For this review, take the finished solid that the model builds, in its own axes (mm). Give positions to 0.01 mm unless a question says otherwise; leave off trailing zeros. Write each loop counter-clockwise with the first axis right and the second up, starting at its lowest first coordinate (ties: lowest second). Pieces come first, ordered by that corner, then holes. Notation, with made-up numbers: (75.5, -0.75) -> (119.5, -0.75) arc R33 ccw to (119.5, 37.25) -> close; hole circle Ø5 at (-10.5, -1). An arc over 180 degrees is marked (long way). Return JSON: item names as keys, results as strings.
from build123d import *

# Parameters (mm, degrees)
F0_W     = 28
F0_H     = 20
F1_DEPTH = 15
F3_D     = 4.4
F4_R     = 6.35
F5_DEPTH = 15.001
F6_R     = 1.5875


with BuildPart() as f1:
    # F0 (on Top) → F1 (new body)
    with BuildSketch(Plane.XY):
        with Locations((14, 10)):
            Rectangle(F0_W, F0_H)
    extrude(amount=F1_DEPTH)

    # F3 (through all)
    with Locations(Plane.XY.offset(15)):
        with Locations((4, 16), (4, 4), (24, 4), (24, 16)):
            Hole(F3_D / 2)

    # F4 (on face) → F5 (cut, through all)
    with BuildSketch(Plane.XY.offset(15)):
        with Locations((14, 10)):
            Circle(F4_R)
    extrude(amount=-F5_DEPTH, mode=Mode.SUBTRACT)

    # F6
    f6_edges = [f1.edges().sort_by_distance(p)[0] for p in [
        (0, 0, 7.5),
        (28, 0, 7.5),
        (28, 20, 7.5),
        (0, 20, 7.5),
    ]]
    fillet(f6_edges, radius=F6_R)


solid = f1.part
1. Add section A-A, the plane x = 14. State the section outline as (y, z) points, plus the area to 4 significant figures.
Results found:
{"outline": "(0, 0) -> (3.65, 0) -> (3.65, 15) -> (0, 15) -> close; (16.35, 0) -> (20, 0) -> (20, 15) -> (16.35, 15) -> close", "area": "109.5 mm²"}
2. The part is to be moulded in two halves that separate along X. For faces 1 (the cylindrical face through (27.52, 19.55, 7.6)), 2 (the flat face through (14, 20, 7)), 3 (the cylindrical face through (20.057, 11.907, 7.605)), say which applies: +X half, -X half, draft (parallel to the pull), parting line (faces both ways), or undercut.
Results found:
{"face 1": "+X half", "face 2": "draft", "face 3": "undercut"}
3. Add section D-D, the plane x = 24. State the section outline as (y, z) points.
Results found:
{"outline": "(0, 0) -> (1.8, 0) -> (1.8, 15) -> (0, 15) -> close; (6.2, 0) -> (13.8, 0) -> (13.8, 15) -> (6.2, 15) -> close; (18.2, 0) -> (20, 0) -> (20, 15) -> (18.2, 15) -> close"}
4. Add section C-C, the plane z = 6.25. Count the separate pieces of the cut face and the enclosed holes in it, plus the area to 3 significant figures.
Results found:
{"separate pieces": "1", "enclosed holes": "5", "area": "370 mm²"}
5. To check wall thickness, follow probe 1 along Y at (x, z) = (4, 11.75); probe 2 along X at (y, z) = (16.5, 11); probe 3 along Y at (x, z) = (3.5, 6.25). State the ranges of each line that lie inside material, in increasing order.
Results found:
{"probe 1": "y = 0 to 1.8, 6.2 to 13.8, 18.2 to 20", "probe 2": "x = 0 to 1.86, 6.14 to 21.86, 26.14 to 28", "probe 3": "y = 0 to 1.86, 6.14 to 13.86, 18.14 to 20"}
6. Add section B-B, the plane y = 10. State the section outline as (x, z) points.
Results found:
{"outline": "(0, 0) -> (7.65, 0) -> (7.65, 15) -> (0, 15) -> close; (20.35, 0) -> (28, 0) -> (28, 15) -> (20.35, 15) -> close"}
7. For pin 1 (5 mm diameter, centred on x = 4, y = 16, fed in from +Z), flat-tipped, find the tip position at first contact; note if it passes through.
Results found:
{"pin 1": "stops at z = 15"}
